```python
from build123d import *

# Parameters (mm, degrees)
CYLINDER007_R     = 1.5
CYLINDER007_DEPTH = 10
CYLINDER006_R     = 1.5
CYLINDER006_DEPTH = 10
CYLINDER005_R     = 1.5
CYLINDER005_DEPTH = 10
CYLINDER004_R     = 1.5
CYLINDER004_DEPTH = 10
CYLINDER001_R     = 8.5
CYLINDER001_DEPTH = 32
FILLET001_R       = 0.6
CYLINDER002_R     = 8.5
CYLINDER002_DEPTH = 3
BOX001_W          = 44.5
BOX001_H          = 44.5
BOX001_DEPTH      = 12.5
BOX_W             = 41.5
BOX_H             = 41.5
BOX_DEPTH         = 32.5
FILLET_R          = 2.5
CHAMFER_SIZE      = 2.5
BOX002_W          = 41.9
BOX002_H          = 41.9
BOX002_DEPTH      = 12.5
CHAMFER001_SIZE   = 4.5
CYLINDER003_R     = 1.25
CYLINDER003_DEPTH = 10
CYLINDER_R        = 2.25
CYLINDER_DEPTH    = 45


with BuildPart() as tornillo020:
    # Cylinder007 → Cylinder007 (new body)
    with BuildSketch(Plane(origin=(-50.4, -6.1, 27), x_dir=(1, 0, 0), z_dir=(0, 0, 1))):
        Circle(CYLINDER007_R)
    extrude(amount=CYLINDER007_DEPTH)


with BuildPart() as tornillo019:
    # Cylinder006 → Cylinder006 (new body)
    with BuildSketch(Plane(origin=(-18.1, -6.1, 27), x_dir=(1, 0, 0), z_dir=(0, 0, 1))):
        Circle(CYLINDER006_R)
    extrude(amount=CYLINDER006_DEPTH)


with BuildPart() as tornillo018:
    # Cylinder005 → Cylinder005 (new body)
    with BuildSketch(Plane(origin=(-50.4, -38.4, 27), x_dir=(1, 0, 0), z_dir=(0, 0, 1))):
        Circle(CYLINDER005_R)
    extrude(amount=CYLINDER005_DEPTH)


with BuildPart() as tornillo017:
    # Cylinder004 → Cylinder004 (new body)
    with BuildSketch(Plane(origin=(-18.1, -38.4, 27), x_dir=(1, 0, 0), z_dir=(0, 0, 1))):
        Circle(CYLINDER004_R)
    extrude(amount=CYLINDER004_DEPTH)


with BuildPart() as fillet001:
    # Cylinder001 → Cylinder001 (new body)
    with BuildSketch(Plane(origin=(-34.2, -22.25, 2), x_dir=(1, 0, 0), z_dir=(0, 0, 1))):
        Circle(CYLINDER001_R)
    extrude(amount=CYLINDER001_DEPTH)

    # Fillet001
    fillet001_edges = [fillet001.edges().sort_by_distance(p)[0] for p in [
        (-42.7, -22.25, 34),
    ]]
    fillet(fillet001_edges, radius=FILLET001_R)


with BuildPart() as cilindro036:
    # Cylinder002 → Cylinder002 (new body)
    with BuildSketch(Plane(origin=(-34.2, -22.25, -1), x_dir=(1, 0, 0), z_dir=(0, 0, 1))):
        Circle(CYLINDER002_R)
    extrude(amount=CYLINDER002_DEPTH)


with BuildPart() as cubo087:
    # Box001 → Box001 (new body)
    with BuildSketch(Plane(origin=(-56, -44, 10), x_dir=(1, 0, 0), z_dir=(0, 0, 1))):
        with Locations((22.25, 22.25)):
            Rectangle(BOX001_W, BOX001_H)
    extrude(amount=BOX001_DEPTH)


with BuildPart() as chamfer_body:
    # Box → Box (new body)
    with BuildSketch(Plane(origin=(-55, -43, 0), x_dir=(1, 0, 0), z_dir=(0, 0, 1))):
        with Locations((20.75, 20.75)):
            Rectangle(BOX_W, BOX_H)
    extrude(amount=BOX_DEPTH)

    # Cut: cut Cubo087
    add(cubo087.part, mode=Mode.SUBTRACT)

    # Fillet
    fillet_edges = [chamfer_body.edges().sort_by_distance(p)[0] for p in [
        (-55, -43, 27.5),
        (-55, -1.5, 27.5),
        (-13.5, -1.5, 27.5),
        (-13.5, -43, 27.5),
    ]]
    fillet(fillet_edges, radius=FILLET_R)

    # Chamfer
    chamfer_edges = [chamfer_body.edges().sort_by_distance(p)[0] for p in [
        (-55, -1.5, 5),
        (-55, -43, 5),
        (-13.5, -1.5, 5),
        (-13.5, -43, 5),
    ]]
    chamfer(chamfer_edges, length=CHAMFER_SIZE)


with BuildPart() as cut001:
    # Box002 → Box002 (new body)
    with BuildSketch(Plane(origin=(-55.2, -43.2, 10), x_dir=(1, 0, 0), z_dir=(0, 0, 1))):
        with Locations((20.95, 20.95)):
            Rectangle(BOX002_W, BOX002_H)
    extrude(amount=BOX002_DEPTH)

    # Chamfer001
    chamfer001_edges = [cut001.edges().sort_by_distance(p)[0] for p in [
        (-55.2, -43.2, 16.25),
        (-55.2, -1.3, 16.25),
        (-13.3, -43.2, 16.25),
        (-13.3, -1.3, 16.25),
    ]]
    chamfer(chamfer001_edges, length=CHAMFER001_SIZE)

    # Fusion: union Chamfer body
    add(chamfer_body.part)

    # Cut001: cut Cilindro036
    add(cilindro036.part, mode=Mode.SUBTRACT)


with BuildPart() as cilindro037:
    # Cylinder003 → Cylinder003 (new body)
    with BuildSketch(Plane(origin=(-34.2, -22.25, 45), x_dir=(1, 0, 0), z_dir=(0, 0, 1))):
        Circle(CYLINDER003_R)
    extrude(amount=CYLINDER003_DEPTH)


with BuildPart() as obj1:
    # Cylinder → Cylinder (new body)
    with BuildSketch(Plane(origin=(-34.2, -22.25, 0), x_dir=(1, 0, 0), z_dir=(0, 0, 1))):
        Circle(CYLINDER_R)
    extrude(amount=CYLINDER_DEPTH)

    # Fusion002: union Fillet001, Cut001, Cilindro037
    add(fillet001.part)
    add(cut001.part)
    add(cilindro037.part)

    # Fusion001: union tornillo020, tornillo019, tornillo018, tornillo017
    add(tornillo020.part)
    add(tornillo019.part)
    add(tornillo018.part)
    add(tornillo017.part)


solid = obj1.part
```
Can you work these out from the model? Positions are in its coordinate system, mm. A direction names the side the tool comes from. Give positions to 0.01 mm unless a question says otherwise; leave off trailing zeros. Loops run counter-clockwise (first coordinate to the right, second up) from the corner with the lowest first, then second, coordinate; pieces in that order, holes last. Notation, with made-up numbers: M -19,41.25 L 25,41.25 A32 ccw 25,77.25 Z; hole C -30.5,-31.5 d3. An arc over 180 degrees is marked long. Use one line per item in the form item = value. Start each with the question number.
(1) On a 3-axis mill with a long thin cutter (end or side, diameter ignored), from which of +Z, -Z, +X, -X, +Y, -Y can I reach the whole of each face in a straight line? I mean faces 1 (the flat face through (-53.4, -41.2, 10)), 2 (the cylindrical face through (-36, -23.6, 39.4)), 3 (the flat face through (-53, -3, 10)), 4 (the flat face through (-55, -23, 5)), 5 (the flat face through (-15.5, -40.9, 16.2)). Say none if no direction works.
(2) I'm going to push flat-ended pins straight in: P1, Ø2, axis at x = -15.5, y = -40.5, coming from the +Z side; P2, Ø5, axis at x = -29, z = 5.5, coming from the +Y side; P3, Ø5, axis at x = -34.5, y = -28, coming from the +Z side. Where does each tip first touch, or does it pass through?
(3) I want a section at C-C, the plane z = 24. Write out the boundary of the cut face in (x, y).
(4) I want a section at B-B, the plane y = -9.5. Write out the boundary of the cut face in (x, z).
(5) Please list where these lines run through material, in increasing order: line 1 (Y direction, x = -34.2, z = 0.4); line 2 (X direction, y = -22.25, z = 0.8); line 3 (Y direction, x = -22, z = 23).
(6) Thinking about a two-plate mould opening in Z: for faces 6 (the cylindrical face through (-16.67, -37.95, 34.72)), 7 (the flat face through (-52.9, -41, 16.2)), 8 (the flat face through (-44, -22, 0)), which applies, released by +Z, released by -Z, zero draft, split by the parting line, or undercut?
(7) I want a section at A-A, the plane x = -23.5. Write out the boundary of the cut face in (y, z).
Worked out:
q1.face_1 = -X, -Y
q1.face_2 = +Z
q1.face_3 = -X, +Y
q1.face_4 = -Z, -X, +Y, -Y
q1.face_5 = +X, -Y
q2.P1 = 32.5
q2.P2 = -1.5
q2.P3 = 34
q3.outline = M -55,-40.5 A2.5 ccw -52.5,-43 L -16,-43 A2.5 ccw -13.5,-40.5 L -13.5,-4 A2.5 ccw -16,-1.5 L -52.5,-1.5 A2.5 ccw -55,-4 Z
q4.outline = M -55.2,10 L -55,10 L -55,0 L -13.5,0 L -13.5,10 L -13.3,10 L -13.3,22.5 L -13.5,22.5 L -13.5,32.5 L -55,32.5 L -55,22.5 L -55.2,22.5 Z
q5.line_1 = -43 to -30.75, -24.5 to -20, -13.75 to -1.5
q5.line_2 = -55 to -42.7, -36.45 to -31.95, -25.7 to -13.5
q5.line_3 = -43 to -1.5
q6.face_6 = zero draft
q6.face_7 = undercut
q6.face_8 = released by -Z
q7.outline = M -43.2,10 L -43,10 L -43,0 L -1.5,0 L -1.5,10 L -1.3,10 L -1.3,22.5 L -1.5,22.5 L -1.5,32.5 L -43,32.5 L -43,22.5 L -43.2,22.5 Z
